```python
from build123d import *

# Parameters (mm, degrees)
CROQUIS2_R              = 1.5875
CROQUIS2_R_2            = 2
CROQUIS2_R_3            = 1.59
CROQUIS2_R_4            = 2.4
SALIENTE_EXTRUIR1_DEPTH = 2


with BuildPart() as part:
    # Croquis2 → Saliente-Extruir1 (new body)
    with BuildSketch(Plane(origin=(0, 0, 0), x_dir=(1, 0, 0), z_dir=(0, 1, 0))):
        with BuildLine():
            Line((-18.114669831, -11.913276785), (-25.665833323, -20.55341124))
            ThreePointArc((-25.665833323, -20.55341124), (-26.522572581, -23.091497469), (-25.333680736, -25.492001591))
            Line((-25.333680736, -25.492001591), (-21.870049663, -28.519089265))
            ThreePointArc((-21.870049663, -28.519089265), (-20.651030144, -29.211556696), (-19.258050197, -29.370070411))
            ThreePointArc((-19.258050197, -29.370070411), (-14.308280019, -31.191358923), (-15.481364298, -26.049259163))
            Line((-15.481364298, -26.049259163), (-9.898337732, -20.139552173))
            ThreePointArc((-9.898337732, -20.139552173), (-6.503541491, -17.615062127), (-2.368704963, -16.720177551))
            Line((-2.368704963, -16.720177551), (2.368704963, -16.720177551))
            ThreePointArc((2.368704963, -16.720177551), (6.503541491, -17.615062127), (9.898337732, -20.139552173))
            Line((9.898337732, -20.139552173), (15.481364298, -26.049259163))
            ThreePointArc((15.481364298, -26.049259163), (14.308280019, -31.191358923), (19.258050197, -29.370070411))
            ThreePointArc((19.258050197, -29.370070411), (20.651030144, -29.211556696), (21.870049663, -28.519089265))
            Line((21.870049663, -28.519089265), (25.333680736, -25.492001591))
            ThreePointArc((25.333680736, -25.492001591), (26.522572581, -23.091497469), (25.665833323, -20.55341124))
            Line((25.665833323, -20.55341124), (18.114669831, -11.913276785))
            ThreePointArc((18.114669831, -11.913276785), (16.282242792, -8.847169319), (15.6443026, -5.332651407))
            Line((15.6443026, -5.332651407), (15.6443026, 5.332651407))
            ThreePointArc((15.6443026, 5.332651407), (16.282242792, 8.847169319), (18.114669831, 11.913276785))
            Line((18.114669831, 11.913276785), (25.665833323, 20.55341124))
            ThreePointArc((25.665833323, 20.55341124), (26.522572581, 23.091497469), (25.333680736, 25.492001591))
            Line((25.333680736, 25.492001591), (21.870049663, 28.519089265))
            ThreePointArc((21.870049663, 28.519089265), (20.516496212, 29.244060494), (18.982893754, 29.319913825))
            ThreePointArc((18.982893754, 29.319913825), (14.561676067, 31.632721836), (14.119221437, 26.662764026))
            Line((14.119221437, 26.662764026), (9.609072603, 20.201124228))
            ThreePointArc((9.609072603, 20.201124228), (6.214276361, 17.676634182), (2.079439834, 16.781749607))
            Line((2.079439834, 16.781749607), (-2.079439834, 16.781749607))
            ThreePointArc((-2.079439834, 16.781749607), (-6.214276361, 17.676634182), (-9.609072603, 20.201124228))
            Line((-9.609072603, 20.201124228), (-14.119221437, 26.662764026))
            ThreePointArc((-14.119221437, 26.662764026), (-13.940786386, 31.181659757), (-18.441858832, 30.742792428))
            ThreePointArc((-18.441858832, 30.742792428), (-19.378360111, 29.807558957), (-20.568781865, 29.229119385))
            ThreePointArc((-20.568781865, 29.229119385), (-21.257437362, 28.943786272), (-21.870049663, 28.519089265))
            Line((-21.870049663, 28.519089265), (-25.333680736, 25.492001591))
            ThreePointArc((-25.333680736, 25.492001591), (-26.522572581, 23.091497469), (-25.665833323, 20.55341124))
            Line((-25.665833323, 20.55341124), (-18.114669831, 11.913276785))
            ThreePointArc((-18.114669831, 11.913276785), (-16.282242792, 8.847169319), (-15.6443026, 5.332651407))
            Line((-15.6443026, 5.332651407), (-15.6443026, -5.332651407))
            ThreePointArc((-15.6443026, -5.332651407), (-16.282242792, -8.847169319), (-18.114669831, -11.913276785))
        make_face()
        with Locations(Location((-16, 29, 0), (0, 0, 270))):
            Circle(CROQUIS2_R, mode=Mode.SUBTRACT)
        with Locations(Location((16, 29, 0), (0, 0, 270))):
            Circle(CROQUIS2_R, mode=Mode.SUBTRACT)
        with Locations(Location((0, 12.497128708, 0), (0, 0, 270))):
            Circle(CROQUIS2_R_2, mode=Mode.SUBTRACT)
        with Locations(Location((0, -12.497128708, 0), (0, 0, 270))):
            Circle(CROQUIS2_R_2, mode=Mode.SUBTRACT)
        with Locations(Location((-15.25, 15.25, 0), (0, 0, 270))):
            Circle(CROQUIS2_R_3, mode=Mode.SUBTRACT)
        with Locations(Location((-15.25, -15.25, 0), (0, 0, 270))):
            Circle(CROQUIS2_R_3, mode=Mode.SUBTRACT)
        with Locations(Location((-20.453154045, 22.873296448, 0), (0, 0, 270))):
            Circle(CROQUIS2_R_4, mode=Mode.SUBTRACT)
        with Locations(Location((20.453154045, 22.873296448, 0), (0, 0, 270))):
            Circle(CROQUIS2_R_4, mode=Mode.SUBTRACT)
        with Locations(Location((20.453154045, -22.873296448, 0), (0, 0, 270))):
            Circle(CROQUIS2_R_4, mode=Mode.SUBTRACT)
        with Locations(Location((-20.453154045, -22.873296448, 0), (0, 0, 270))):
            Circle(CROQUIS2_R_4, mode=Mode.SUBTRACT)
        with Locations(Location((15.25, -15.25, 0), (0, 0, 270))):
            Circle(CROQUIS2_R_3, mode=Mode.SUBTRACT)
        with Locations(Location((15.25, 15.25, 0), (0, 0, 270))):
            Circle(CROQUIS2_R_3, mode=Mode.SUBTRACT)
        with Locations(Location((-16, -29, 0), (0, 0, 270))):
            Circle(CROQUIS2_R, mode=Mode.SUBTRACT)
        with Locations(Location((16, -29, 0), (0, 0, 270))):
            Circle(CROQUIS2_R, mode=Mode.SUBTRACT)
        with BuildLine():
            Line((-8.997091839, 11.368814033), (-10.997834751, 9.446969084))
            ThreePointArc((-10.997834751, 9.446969084), (-11.601593103, 7.79748332), (-10.670982222, 6.30775488))
            Line((-10.670982222, 6.30775488), (-5.87110313, 3.313187619))
            ThreePointArc((-5.87110313, 3.313187619), (-3.426979279, 3.567667883), (-3.074423593, 5.999581964))
            Line((-3.074423593, 5.999581964), (-5.873559772, 10.915994174))
            ThreePointArc((-5.873559772, 10.915994174), (-7.324662306, 11.905756202), (-8.997091839, 11.368814033))
        make_face(mode=Mode.SUBTRACT)
        with BuildLine():
            Line((5.873559772, 10.915994174), (3.074423593, 5.999581964))
            ThreePointArc((3.074423593, 5.999581964), (3.426979279, 3.567667883), (5.87110313, 3.313187619))
            Line((5.87110313, 3.313187619), (10.670982222, 6.30775488))
            ThreePointArc((10.670982222, 6.30775488), (11.601593103, 7.79748332), (10.997834751, 9.446969084))
            Line((10.997834751, 9.446969084), (8.997091839, 11.368814033))
            ThreePointArc((8.997091839, 11.368814033), (7.324662306, 11.905756202), (5.873559772, 10.915994174))
        make_face(mode=Mode.SUBTRACT)
        with BuildLine():
            Line((8.997091839, -11.368814033), (10.997834751, -9.446969084))
            ThreePointArc((10.997834751, -9.446969084), (11.601593103, -7.79748332), (10.670982222, -6.30775488))
            Line((10.670982222, -6.30775488), (5.87110313, -3.313187619))
            ThreePointArc((5.87110313, -3.313187619), (3.426979279, -3.567667883), (3.074423593, -5.999581964))
            Line((3.074423593, -5.999581964), (5.873559772, -10.915994174))
            ThreePointArc((5.873559772, -10.915994174), (7.324662306, -11.905756202), (8.997091839, -11.368814033))
        make_face(mode=Mode.SUBTRACT)
        with BuildLine():
            Line((-5.873559772, -10.915994174), (-3.074423593, -5.999581964))
            ThreePointArc((-3.074423593, -5.999581964), (-3.426979279, -3.567667883), (-5.87110313, -3.313187619))
            Line((-5.87110313, -3.313187619), (-10.670982222, -6.30775488))
            ThreePointArc((-10.670982222, -6.30775488), (-11.601593103, -7.79748332), (-10.997834751, -9.446969084))
            Line((-10.997834751, -9.446969084), (-8.997091839, -11.368814033))
            ThreePointArc((-8.997091839, -11.368814033), (-7.324662306, -11.905756202), (-5.873559772, -10.915994174))
        make_face(mode=Mode.SUBTRACT)
    extrude(amount=SALIENTE_EXTRUIR1_DEPTH)


solid = part.part
```
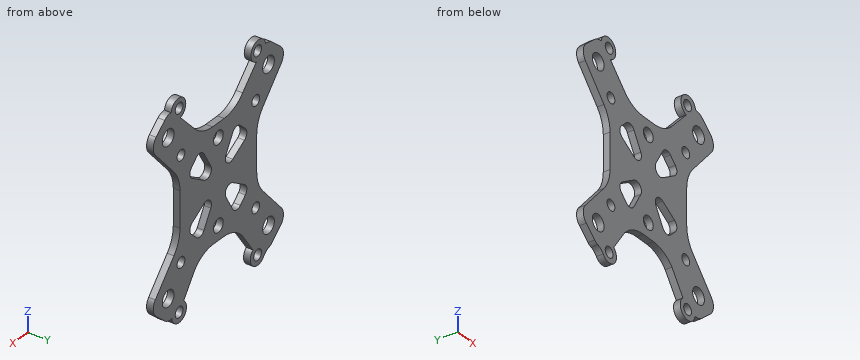
Part model, mm, in its own coordinate system. Round coordinates to 2 decimals unless told otherwise and drop trailing zeros. Write each loop counter-clockwise with the first axis right and the second up, starting at its lowest first coordinate (ties: lowest second). Pieces come first, ordered by that corner, then holes. Notation, with made-up numbers: M -31.75,-3 L -9.75,-3 A26 cw -9.75,18 Z; hole C 63,-13.5 d9. An arc over 180 degrees is marked long. One line per question, with ' | ' between items.
(1) Saw through at A-A on z = -19. Write the cut outline in (x, y).
Answer key:
outline: M -24.31,0 L -8.36,0 L -8.36,2 L -24.31,2 Z; M 8.36,0 L 24.31,0 L 24.31,2 L 8.36,2 Z
(2) Saw through at C-C on z = 15.25. Write the cut outline in (x, y).
Answer key:
outline: M -21.03,0 L -16.84,0 L -16.84,2 L -21.03,2 Z; M -13.66,0 L 13.66,0 L 13.66,2 L -13.66,2 Z; M 16.84,0 L 21.03,0 L 21.03,2 L 16.84,2 Z
(3) Saw through at D-D on y = 1.45. Count the separate pieces of the cut face and the enclosed holes in it, then the cut area to 3 significant figures.
Answer key:
separate pieces: 1 | enclosed holes: 18 | area: 1,520 mm^2
(4) Pin check, flat tip, straight feed: pin 1 (1 mm diameter, centred on x = 0, y = 0.5, fed in from -Z). Stop position of the tip, or through.
Answer key:
pin 1: stops at z = -16.78
(5) Saw through at B-B on x = -4.5. Write the cut outline in (y, z).
Answer key:
outline: M 0,-17.08 L 2,-17.08 L 2,-8.5 L 0,-8.5 Z; M 0,-3.03 L 2,-3.03 L 2,3.03 L 0,3.03 Z; M 0,8.5 L 2,8.5 L 2,16.95 L 0,16.95 Z
(6) Probe line 1 along X through (y, z) = (1.45, 21); line 2 along X through (y, z) = (1.1, -29); line 3 along X through (y, z) = (0.8, 15.25). List the from-to ranges inside material, lowest first.
Answer key:
line 1: x = -26 to -21.95, -18.95 to -10.71, 10.71 to 18.95, 21.95 to 26 | line 2: x = -21.15 to -17.59, -14.41 to -13, 13 to 14.41, 17.59 to 21.15 | line 3: x = -21.03 to -16.84, -13.66 to 13.66, 16.84 to 21.03
